Geometry check sheet. Reference: the model listing, model coordinates, mm. A direction names the side the tool comes from. Round coordinates to 2 decimals unless told otherwise and drop trailing zeros. Write each loop counter-clockwise with the first axis right and the second up, starting at its lowest first coordinate (ties: lowest second). Pieces come first, ordered by that corner, then holes. Notation, with made-up numbers: (-18, -39.5) - (18, -39.5) arc R25 cw to (18, -11.5) - close; hole circle Ø2 at (22.5, -0.5). An arc over 180 degrees is marked (long way). Return JSON: item names as keys, results as strings.
```python
from build123d import *

# Parameters (mm, degrees)
SKETCH1_W           = 146
SKETCH1_H           = 20
BOSS_EXTRUDE1_DEPTH = 30
SKETCH2_R           = 3.25
CUT_EXTRUDE1_DEPTH  = 30
SKETCH3_R           = 7.475
CUT_EXTRUDE2_DEPTH  = 150.385407587
SKETCH4_R           = 5.7225
CUT_EXTRUDE3_DEPTH  = 15


with BuildPart() as part:
    # Sketch1 → Boss-Extrude1 (new body)
    with BuildSketch(Plane(origin=(0, 0, 0), x_dir=(1, 0, 0), z_dir=(0, 1, 0))):
        Rectangle(SKETCH1_W, SKETCH1_H)
    extrude(amount=BOSS_EXTRUDE1_DEPTH)

    # Sketch2 → Cut-Extrude1 (cut)
    with BuildSketch(Plane.XY.offset(10)):
        with Locations((-36, 24)):
            Circle(SKETCH2_R)
        with Locations((36, 24)):
            Circle(SKETCH2_R)
    extrude(amount=-CUT_EXTRUDE1_DEPTH, mode=Mode.SUBTRACT)

    # Sketch3 → Cut-Extrude2 (cut, through all)
    with BuildSketch(Plane.ZY.offset(73)):
        with Locations((0, 11)):
            Circle(SKETCH3_R)
    extrude(amount=-CUT_EXTRUDE2_DEPTH, mode=Mode.SUBTRACT)

    # Sketch4 → Cut-Extrude3 (cut)
    with BuildSketch(Plane(origin=(0, 30, 0), x_dir=(1, 0, 0), z_dir=(0, 1, 0))):
        with Locations(Location((-54, 0, 0), (0, 0, 270))):
            Circle(SKETCH4_R)
        with Locations(Location((-18, 0, 0), (0, 0, 270))):
            Circle(SKETCH4_R)
        with Locations(Location((18, 0, 0), (0, 0, 270))):
            Circle(SKETCH4_R)
        with Locations(Location((54, 0, 0), (0, 0, 270))):
            Circle(SKETCH4_R)
    extrude(amount=-CUT_EXTRUDE3_DEPTH, mode=Mode.SUBTRACT)


solid = part.part
```
(1) Gauge pin test, flat ends, axial feed: pin 1 (12 mm diameter, centred on y = 11, z = 0, fed in from -X); pin 2 (7 mm diameter, centred on x = 54, z = 0, fed in from +Y); pin 3 (9 mm diameter, centred on x = -18, z = 0, fed in from +Y). Record the tip position at first contact, or that the pin passes through.
Response values:
{"pin 1": "passes through", "pin 2": "stops at y = 4.4", "pin 3": "stops at y = 5.03"}
(2) Access from +Z, -Z, +X, -X, +Y, -Y to the whole of each face (thin tool, end or side, straight path). Record for faces 1 (the face through (-1, 15, -10)), 2 (the face through (19.719, 23.004, 5.458)).
Response values:
{"face 1": "-Z, +X, -X, +Y, -Y", "face 2": "+Y"}
(3) Material ranges on line 1 along X through (y, z) = (19.5, 0); line 2 along Z through (x, y) = (18, 22.5); line 3 along Y through (x, z) = (36, -5.5), recorded low to high. Write a range as [from, to].
Response values:
{"line 1": "x = [-73, -59.72], [-48.28, -23.72], [-12.28, 12.28], [23.72, 48.28], [59.72, 73]", "line 2": "z = [-10, -5.72], [5.72, 10]", "line 3": "y = [0, 5.94], [16.06, 20.75], [27.25, 30]"}
(4) Section check A-A, the plane x = 36. Enter the section's corners in (y, z) (3 decimals), plus the area to 3 significant figures.
Response values:
{"outline": "(0, -10) - (20.75, -10) - (20.75, 10) - (0, 10) - close; (27.25, -10) - (30, -10) - (30, 10) - (27.25, 10) - close; hole circle Ø14.95 at (11, 0)", "area": "294 mm^2"}
(5) Section check D-D, the plane y = 11. Enter the section's corners in (x, z) (3 decimals), plus the area to 3 significant figures.
Response values:
{"outline": "(-73, -10) - (73, -10) - (73, -7.475) - (-73, -7.475) - close; (-73, 7.475) - (73, 7.475) - (73, 10) - (-73, 10) - close", "area": "737 mm^2"}
(6) Section check B-B, the plane y = 24. Give the number of separate pieces and of enclosed holes in the cut face, plus the area to 3 significant figures.
Response values:
{"separate pieces": "3", "enclosed holes": "4", "area": "2,250 mm^2"}
(7) Release check for a two-part mould opening along X. For faces 3 (the face through (-32.998, 22.755, 0.14)), 4 (the face through (-73, 18, 5)), 5 (the face through (73, 18, 5)), 6 (the face through (-1, 30, 0)) record: pulls with the +X half, pulls with the -X half, needs draft (parallel to the pull), parting line crosses it, or undercut.
Response values:
{"face 3": "undercut", "face 4": "pulls with the -X half", "face 5": "pulls with the +X half", "face 6": "needs draft"}
